Work out the finished part from the listing and answer in its coordinate system (mm). A direction names the side the tool comes from. Round coordinates to 2 decimals unless told otherwise and drop trailing zeros. Write each loop counter-clockwise with the first axis right and the second up, starting at its lowest first coordinate (ties: lowest second). Pieces come first, ordered by that corner, then holes. Notation, with made-up numbers: M 33,-21 L 78,-21 A8 cw 78,-11 Z; hole C -13.75,85 d3. An arc over 180 degrees is marked long. Answer in a Markdown table with one row per item.
```python
from build123d import *
from OCP.BRepFilletAPI import BRepFilletAPI_MakeFillet

# Parameters (mm, degrees)
SKETCH1_W           = 19
SKETCH1_H           = 30.5
SKETCH1_R           = 0.5
PCB_DEPTH           = 1.6
PCB_FILLET_R        = 3
USB_START           = 1.6
SKETCH1_3_W         = 9
SKETCH1_3_H         = 7.05
SKETCH1_3_H_2       = 0.25
USB_C_DEPTH         = 3.3
USB_C_FILLET_R      = 1.65
POWER_START         = 1.6
SKETCH1_4_W         = 2.5
SKETCH1_4_H         = 7.4
POWER_JUMPERS_DEPTH = 8.6
UART_START          = 1.6
SKETCH1_5_W         = 13
SKETCH1_5_H         = 2.5
UART_TO_BOARD_DEPTH = 4.5
SKETCH3_W           = 13
SKETCH3_H           = 2.5
UART_PINS_DEPTH     = 5.5
UART_FILLET_R1      = 1.5
UART_FILLET_R2      = 0.5
LPATTERN1_OUTLINE_R = 0.5
LPATTERN1_DEPTH     = 1.6


# Read off the part's stored shape, not the designer's step: LPattern1
with BuildPart() as part:
    # Sketch1 → PCB (new body)
    with BuildSketch(Plane(origin=(0, 0, 0), x_dir=(1, 0, 0), z_dir=(0, 1, 0))):
        Rectangle(SKETCH1_W, SKETCH1_H)
        with Locations(Location((7.75, 0.95, 0), (0, 0, 270))):
            Circle(SKETCH1_R, mode=Mode.SUBTRACT)
    extrude(amount=PCB_DEPTH)

    # PCB Fillet
    pcb_fillet_edges = [part.edges().sort_by_distance(p)[0] for p in [
        (9.5, 0.8, -15.25),
        (9.5, 0.8, 15.25),
        (-9.5, 0.8, 15.25),
        (-9.5, 0.8, -15.25),
    ]]
    fillet(pcb_fillet_edges, radius=PCB_FILLET_R)

    # Sketch1<3> → USB C (add)
    with BuildSketch(Plane(origin=(0, 0, 0), x_dir=(1, 0, 0), z_dir=(0, 1, 0)).offset(USB_START)):
        with Locations((0, 11.725)):
            Rectangle(SKETCH1_3_W, SKETCH1_3_H)
        with Locations((0, 15.375)):
            Rectangle(SKETCH1_3_W, SKETCH1_3_H_2)
    extrude(amount=USB_C_DEPTH)

    # USB C Fillet
    usb_c_fillet_edges = [part.edges().sort_by_distance(p)[0] for p in [
        (-4.5, 4.9, -11.85),
        (-4.5, 1.6, -15.375),
        (4.5, 4.9, -11.85),
        (4.5, 1.6, -15.375),
    ]]
    fillet(usb_c_fillet_edges, radius=USB_C_FILLET_R - 0.0001)  # a hair under: the kernel refuses the full size

    # Sketch1<4> → Power Jumpers (add)
    with BuildSketch(Plane(origin=(0, 0, 0), x_dir=(1, 0, 0), z_dir=(0, 1, 0)).offset(POWER_START)):
        with Locations((-8, -0.45)):
            Rectangle(SKETCH1_4_W, SKETCH1_4_H)
    extrude(amount=POWER_JUMPERS_DEPTH)

    # Sketch1<5> → UART To Board (add)
    with BuildSketch(Plane(origin=(0, 0, 0), x_dir=(1, 0, 0), z_dir=(0, 1, 0)).offset(UART_START)):
        with Locations((0, -13.5)):
            Rectangle(SKETCH1_5_W, SKETCH1_5_H)
    extrude(amount=UART_TO_BOARD_DEPTH)

    # Sketch3 → UART Pins (add)
    with BuildSketch(Plane.XY.offset(14.75)):
        with Locations((0, 4.85)):
            Rectangle(SKETCH3_W, SKETCH3_H)
    extrude(amount=UART_PINS_DEPTH)

    # UART Fillet: one fillet with a radius per group of edges: ONE call of the kernel's fillet builder (fillet() takes one radius for all edges)
    uart_fillet_edges_1 = [part.edges().sort_by_distance(p)[0] for p in [
        (0, 6.1, 12.25),
    ]]
    uart_fillet_edges_2 = [part.edges().sort_by_distance(p)[0] for p in [
        (0, 3.6, 14.75),
    ]]
    uart_fillet = BRepFilletAPI_MakeFillet(part.part.solid().wrapped)
    for e in uart_fillet_edges_1:
        uart_fillet.Add(UART_FILLET_R1, e.wrapped)
    for e in uart_fillet_edges_2:
        uart_fillet.Add(UART_FILLET_R2, e.wrapped)
    add(Compound.cast(uart_fillet.Shape()), mode=Mode.REPLACE)

    # LPattern1 outline → LPattern1 (cut)
    with BuildSketch(Plane(origin=(0, 0, 0), x_dir=(1, 0, 0), z_dir=(0, 1, 0))):
        with Locations((7.75, -6.55)):
            Circle(LPATTERN1_OUTLINE_R)
        with Locations((7.75, -4.05)):
            Circle(LPATTERN1_OUTLINE_R)
        with Locations((7.75, -1.55)):
            Circle(LPATTERN1_OUTLINE_R)
    extrude(amount=LPATTERN1_DEPTH, mode=Mode.SUBTRACT)


solid = part.part
```
1. Consider line 1 along X through (y, z) = (3.5, 2); line 2 along Y through (x, z) = (3.75, -3); line 3 along Z through (x, y) = (6, 4.75). Determine where each line is inside the solid, lowest interval first. Write a range as from..to.
Calculated:
| item | result |
|---|---|
| line 1 | x = -9.25..-6.75 |
| line 2 | y = 0..1.6 |
| line 3 | z = 12.26..20.25 |
2. The part is cut by section A-A (z = 6.55). Determine the outline of the cut face in (x, y).
Calculated:
| item | result |
|---|---|
| outline | M -9.5,0 L 7.25,0 L 7.25,1.6 L -9.5,1.6 Z; M 8.25,0 L 9.5,0 L 9.5,1.6 L 8.25,1.6 Z |
3. Given pin 1 (0.5 mm diameter, centred on x = -1, y = 1, fed in from +Z); pin 2 (1.3 mm diameter, centred on y = 4.5, z = 14.5, fed in from -X); pin 3 (4.5 mm diameter, centred on x = 1.5, z = -11.5, fed in from +Y), each flat-ended and moving along its own axis, determine where each tip first touches the part or whether it passes through.
Calculated:
| item | result |
|---|---|
| pin 1 | stops at z = 15.25 |
| pin 2 | stops at x = -6.5 |
| pin 3 | stops at y = 4.9 |
4. A tool of negligible diameter and unlimited length cuts with its end or side. For faces 1 (the flat face through (-8, 6, 4.15)), 2 (the flat face through (0, 1, 15.25)), 3 (the flat face through (-6.5, 4, 15)), 4 (the flat face through (-6.75, 6, 1)), from which of +Z, -Z, +X, -X, +Y, -Y can it reach the whole face along a straight path? Write none if from no direction.
Calculated:
| item | result |
|---|---|
| face 1 | +Z, +X, -X, +Y |
| face 2 | +Z, +X, -X, -Y |
| face 3 | +Z, -Z, -X, +Y |
| face 4 | +Z, -Z, +X, +Y |
5. The part is cut by section D-D (z = 1.55). Determine the outline of the cut face in (x, y).
Calculated:
| item | result |
|---|---|
| outline | M -9.5,0 L 7.25,0 L 7.25,1.6 L -6.75,1.6 L -6.75,10.2 L -9.25,10.2 L -9.25,1.6 L -9.5,1.6 Z; M 8.25,0 L 9.5,0 L 9.5,1.6 L 8.25,1.6 Z |
6. Determine the mould class of faces 5 (the flat face through (-9.5, 1, 0)), 6 (the flat face through (0, 3, 12.25)), 7 (the cylindrical face through (7.262, 0.789, -1.058)) for opening direction X: released by +X, released by -X, zero draft, split by the parting line, or undercut.
Calculated:
| item | result |
|---|---|
| face 5 | released by -X |
| face 6 | zero draft |
| face 7 | undercut |
7. The part is cut by section B-B (y = 1). Determine the outline of the cut face in (x, z), plus the area to 3 significant figures.
Calculated:
| item | result |
|---|---|
| outline | M -9.5,-12.25 A3 ccw -6.5,-15.25 L 6.5,-15.25 A3 ccw 9.5,-12.25 L 9.5,12.25 A3 ccw 6.5,15.25 L -6.5,15.25 A3 ccw -9.5,12.25 Z; hole C 7.75,-0.95 d1; hole C 7.75,1.55 d1; hole C 7.75,4.05 d1; hole C 7.75,6.55 d1 |
| area | 569 mm² |
8. The part is cut by section C-C (x = -2.5). Determine the outline of the cut face in (y, z), plus the area to 3 significant figures.
Calculated:
| item | result |
|---|---|
| outline | M 0,-15.25 L 1.6,-15.25 L 1.6,-15.5 L 4.9,-15.5 L 4.9,-8.2 L 1.6,-8.2 L 1.6,12.25 L 4.6,12.25 A1.5 ccw 6.1,13.75 L 6.1,20.25 L 3.6,20.25 L 3.6,15.25 A0.5 cw 3.1,14.75 L 1.6,14.75 L 1.6,15.25 L 0,15.25 Z |
| area | 97.5 mm² |
